Work out the finished part from the listing and answer in its coordinate system (mm). Give positions to 0.01 mm unless a question says otherwise; leave off trailing zeros. Write each loop counter-clockwise with the first axis right and the second up, starting at its lowest first coordinate (ties: lowest second). Pieces come first, ordered by that corner, then holes. Notation, with made-up numbers: (48, -38.75) - (86, -38.75) arc R32 ccw to (86, -8.75) - close; hole circle Ø2 at (28.5, -32). An arc over 180 degrees is marked (long way). Write item = value, one per line.
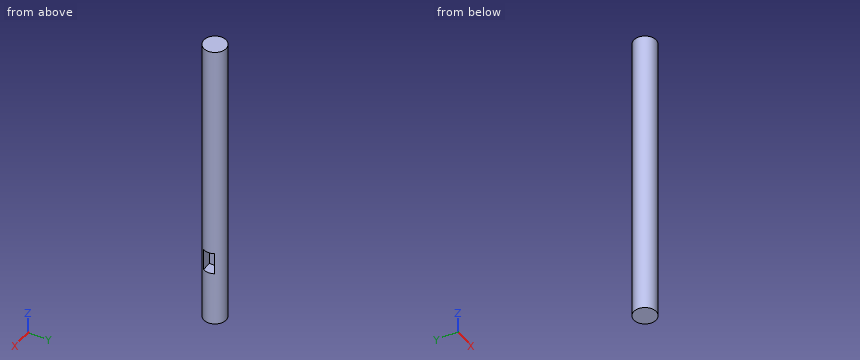
from build123d import *

# Parameters (mm, degrees)
F0_R     = 25.4
F1_DEPTH = 228.6
F2_DEPTH = 457.2
F5_W     = 25.4
F5_H     = 50.8
F6_DEPTH = 25.4


with BuildPart() as f1:
    # F0 (on Top) → F1 (new body)
    with BuildSketch(Plane.XY):
        Circle(F0_R)
    extrude(amount=F1_DEPTH)

    # F0 (on Top) → F2 (join)
    with BuildSketch(Plane.XY):
        Circle(F0_R)
    extrude(amount=-F2_DEPTH)

    # F5 (on face) → F6 (cut)
    with BuildSketch(Plane.YZ.offset(25.4)):
        with Locations((0, -305.080473)):
            Rectangle(F5_W, F5_H)
    extrude(amount=-F6_DEPTH, mode=Mode.SUBTRACT)


solid = f1.part
1. Find section D-D, the plane z = -322. Give the vertices of the cut face in (x, y), then the cut area to 3 significant figures.
Solution:
outline = (0, -12.7) - (0, 12.7) - (22, 12.7) arc R25.4 ccw (long way) to (22, -12.7) - close
area = 1,410 mm^2
2. Find section B-B, the plane z = -213. Give the vertices of the cut face in (x, y).
Solution:
outline = circle Ø50.8 at (0, 0)
3. Find section C-C, the plane y = 6.5. Give the vertices of the cut face in (x, z).
Solution:
outline = (-24.55, -457.2) - (24.55, -457.2) - (24.55, -330.48) - (0, -330.48) - (0, -279.68) - (24.55, -279.68) - (24.55, 228.6) - (-24.55, 228.6) - close
4. Straight lines are drawn through the part: line 1 (Z direction, x = 8, y = 9.5); line 2 (Y direction, x = 18.5, z = -302); line 3 (X direction, y = 2.5, z = 135). For each, find the intervals that lie inside material, in ascending order.
Solution:
line_1 = -457.2 to -330.48, -279.68 to 228.6
line_2 = -17.4 to -12.7, 12.7 to 17.4
line_3 = -25.28 to 25.28
5. Find section A-A, the plane x = 13.5. Give the vertices of the cut face in (y, z), then the cut area to 3 significant figures.
Solution:
outline = (-21.52, -457.2) - (21.52, -457.2) - (21.52, 228.6) - (-21.52, 228.6) - close; hole (-12.7, -330.48) - (12.7, -330.48) - (12.7, -279.68) - (-12.7, -279.68) - close
area = 28,200 mm^2
6. Given pin 1 (2 mm diameter, centred on y = -3, z = -241, fed in from -X); pin 2 (12 mm diameter, centred on y = -12, z = -247, fed in from +X); pin 3 (2 mm diameter, centred on y = -20, z = -198, fed in from +X), each flat-ended and moving along its own axis, determine where each tip first touches the part or whether it passes through.
Solution:
pin_1 = -25.32
pin_2 = 24.68
pin_3 = 16.86
